from build123d import *

# Parameters (mm, degrees)
F0_W     = 488.089332
F0_H     = 428.058626
F0_W_2   = 408.089332
F0_H_2   = 341.250144
F1_DEPTH = 100
F2_R     = 50
F3_R     = 25


with BuildPart() as f1:
    # F0 (on Top) → F1 (new body)
    with BuildSketch(Plane.XY):
        Rectangle(F0_W, F0_H)
        Rectangle(F0_W_2, F0_H_2, mode=Mode.SUBTRACT)
    extrude(amount=F1_DEPTH)

    # F2
    f2_edges = [f1.edges().sort_by_distance(p)[0] for p in [
        (-244.044666, 214.029313, 50),
        (-244.044666, -214.029313, 50),
        (-204.044666, 170.625072, 50),
    ]]
    fillet(f2_edges, radius=F2_R)

    # F3
    f3_edges = [f1.edges().sort_by_distance(p)[0] for p in [
        (-204.044666, -170.625072, 50),
    ]]
    fillet(f3_edges, radius=F3_R)


solid = f1.part
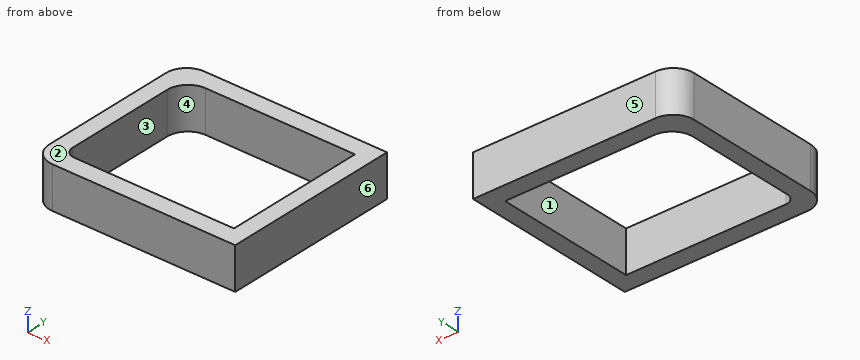
Check sheet for the modelled part. Datum: model origin and axes. Units: mm. Face numbers are marked on the shaded views. A direction names the side the tool comes from. Give positions to 0.01 mm unless a question says otherwise; leave off trailing zeros. Write each loop counter-clockwise with the first axis right and the second up, starting at its lowest first coordinate (ties: lowest second). Pieces come first, ordered by that corner, then holes. Notation, with made-up numbers: (38, 31) -> (57, 31) arc R29 ccw to (57, 62) -> close; hole circle Ø2 at (46, 40.25). An arc over 180 degrees is marked (long way). One line per item, written item: value. Start each with the question number.
Item 1: Tool access check on the marked faces 1 and 2. Record the directions out of +Z, -Z, +X, -X, +Y, -Y that give a thin tool (end or side, any length) a straight path to the whole face; none if there is none.
Item 2: Draft check along Y on the marked faces 3, 4, 5 and 6. Enter one of: +Y half, -Y half, draft (parallel to the pull), parting line (faces both ways), or undercut.
Item 3: Section check C-C on z = 18.5. Record the cut outline in (x, y), then the cut area to 3 significant figures.
Item 4: Section check D-D on x = -214. Record the cut outline in (y, z), then the cut area to 3 significant figures.
Item 5: Material ranges on probe 1 along Y at (x, z) = (65.5, 65.5); probe 2 along X at (y, z) = (19.5, 73.5); probe 3 along Y at (x, z) = (-179, 43.5), recorded low to high. Write a range as from..to.
Item 6: Section check B-B on x = -33.5. Record the cut outline in (y, z), then the cut area to 3 significant figures.
Item 7: Section check A-A on y = 29. Record the cut outline in (x, z), then the cut area to 3 significant figures.
Results list:
1. face 1: +Z, -Z
1. face 2: +Z, +X, -X, +Y, -Y
2. face 3: undercut
2. face 4: undercut
2. face 5: +Y half
2. face 6: draft
3. outline: (-244.04, -164.03) arc R50 ccw to (-194.04, -214.03) -> (244.04, -214.03) -> (244.04, 214.03) -> (-194.04, 214.03) arc R50 ccw to (-244.04, 164.03) -> close; hole (-204.04, -145.63) arc R25 ccw to (-179.04, -170.63) -> (204.04, -170.63) -> (204.04, 170.63) -> (-154.04, 170.63) arc R50 ccw to (-204.04, 120.63) -> close
3. area: 69,300 mm²
4. outline: (-209.87, 0) -> (209.87, 0) -> (209.87, 100) -> (-209.87, 100) -> close
4. area: 42,000 mm²
5. probe 1: -214.03..-170.63, 170.63..214.03
5. probe 2: -244.04..-204.04, 204.04..244.04
5. probe 3: -214.03..-170.63, 163.95..214.03
6. outline: (-214.03, 0) -> (-170.63, 0) -> (-170.63, 100) -> (-214.03, 100) -> close; (170.63, 0) -> (214.03, 0) -> (214.03, 100) -> (170.63, 100) -> close
6. area: 8,680 mm²
7. outline: (-244.04, 0) -> (-204.04, 0) -> (-204.04, 100) -> (-244.04, 100) -> close; (204.04, 0) -> (244.04, 0) -> (244.04, 100) -> (204.04, 100) -> close
7. area: 8,000 mm²
